The figure shows three views and two pictorial views of one solid part (mm, origin at its lowest corner). Answer the questions. A direction names the side the tool comes from. Round coordinates to 2 decimals unless told otherwise and drop trailing zeros. Order: outer loops, then holes, each group sorted by start corner. A loop starts at its lowest first (then second) coordinate and runs counter-clockwise, first axis right, second up. Notation, with made-up numbers: (-0.5, 19) -> (5.5, 19) arc R18 cw to (5.5, 23) -> close; hole circle Ø11 at (52, 75.25). An arc over 180 degrees is marked (long way). Answer as a JSON object with one key per item and string values. Group by question number.
Item 1: Section D-D, the plane x = 39.5 is taken. Write down the section's boundary in (y, z), plus the area to 3 significant figures.
Item 2: Consider probe 1 along Z at (x, y) = (20.25, 11); probe 2 along Z at (x, y) = (13.5, 43.5); probe 3 along Y at (x, z) = (8, 36.5). Determine where each line is inside the solid, lowest interval first. Write a range as from..to.
Item 3: For the marked faces 1, 2, 3, 4 and 5, determine the directions among +Z, -Z, +X, -X, +Y, -Y from which every point of the face is accessible in a straight line to the end or side of a thin tool.
Item 4: Section B-B, the plane z = 10 is taken. Write down the section's boundary in (x, y).
Item 5: Given P1, Ø6, axis at x = 8.5, z = 13, coming from the +Y side; P2, Ø4, axis at y = 11, z = 31, coming from the +X side; P3, Ø10.5, axis at y = 17.5, z = 12, coming from the -X side, each flat-ended and moving along its own axis, determine where each tip first touches the part or whether it passes through.
Item 6: Section A-A, the plane y = 26 is taken. Write down the section's boundary in (x, z).
Item 7: Section C-C, the plane y = 18 is taken. Write down the section's boundary in (x, z).
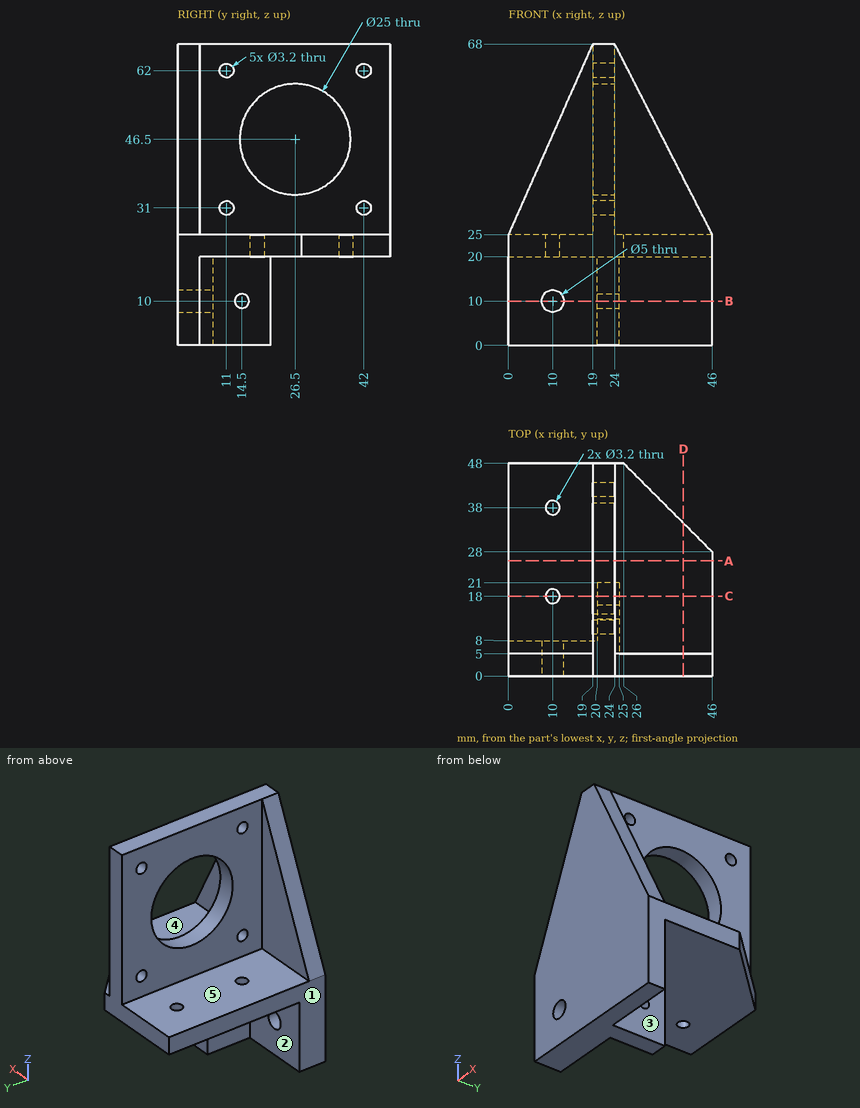
Values found:
{
 "1": {"outline": "(0, 0) -> (5, 0) -> (5, 20) -> (34.5, 20) -> (34.5, 25) -> (5, 25) -> (5, 37.7) -> (0, 37.7) -> close", "area": "336 mm2"},
 "2": {"probe 1": "0..29.4, 32.6..60.4, 63.6..68", "probe 2": "20..25", "probe 3": "0..5"},
 "3": {"face 1": "+Z, -Z, -X, +Y, -Y", "face 2": "-Z, -X, +Y", "face 3": "-Z, +X, +Y", "face 4": "+Z, +X, +Y", "face 5": "+Z, -X, +Y"},
 "4": {"outline": "(0, 0) -> (7.5, 0) -> (7.5, 8) -> (0, 8) -> close; (12.5, 0) -> (46, 0) -> (46, 5) -> (25, 5) -> (25, 12.9) -> (20, 12.9) -> (20, 8) -> (12.5, 8) -> close; (20, 16.1) -> (25, 16.1) -> (25, 21) -> (20, 21) -> close"},
 "5": {"P1": "y = 8", "P2": "x = 24", "P3": "x = 20"},
 "6": {"outline": "(0, 20) -> (46, 20) -> (46, 25) -> (24, 25) -> (24, 34.01) -> (19, 34.01) -> (19, 25) -> (0, 25) -> close; (19, 58.99) -> (24, 58.99) -> (24, 68) -> (19, 68) -> close"},
 "7": {"outline": "(0, 20) -> (8.4, 20) -> (8.4, 25) -> (0, 25) -> close; (11.6, 20) -> (20, 20) -> (20, 0) -> (25, 0) -> (25, 20) -> (46, 20) -> (46, 25) -> (24, 25) -> (24, 37.33) -> (19, 37.33) -> (19, 25) -> (11.6, 25) -> close; (19, 55.67) -> (24, 55.67) -> (24, 68) -> (19, 68) -> close"}
}
